```python
from build123d import *

# Parameters (mm, degrees)
BOSS_EXTRUDE1_DEPTH = 37.592
FILLET1_R           = 12.7
FILLET2_R           = 50.8
FILLET3_R           = 12.7
SCALE1_SCALE        = 0.05


with BuildPart() as part:
    # Sketch1 → Boss-Extrude1 (new body)
    with BuildSketch(Plane.XY):
        with BuildLine():
            Line((0, 109.420372667), (250.19, 109.420372667))
            ThreePointArc((250.19, 109.420372667), (267.97, 91.640372667), (250.19, 73.860372667))
            Line((250.19, 73.860372667), (237.49, 73.860372667))
            Line((237.49, 73.860372667), (237.49, 23.060372667))
            Line((237.49, 23.060372667), (250.19, 23.060372667))
            ThreePointArc((250.19, 23.060372667), (267.97, 5.280372667), (250.19, -12.499627333))
            ThreePointArc((250.19, -12.499627333), (146.843102498, -20.027410993), (44.744230284, -37.721168163))
            ThreePointArc((44.744230284, -37.721168163), (-1.227067533, -59.631780483), (17.441932467, -12.25136687))
            ThreePointArc((17.441932467, -12.25136687), (107.033415037, 14.717722357), (200.152, 23.822372667))
            Line((200.152, 23.822372667), (200.152, 72.082372667))
            Line((200.152, 72.082372667), (-75.968392762, 72.082372667))
            Line((-75.968392762, 72.082372667), (-75.968392762, 21.282372667))
            Line((-75.968392762, 21.282372667), (-96.52, 21.282372667))
            Line((-96.52, 21.282372667), (-170.457211488, 45.010876589))
            Line((-170.457211488, 45.010876589), (-170.457211488, 77.522876589))
            Line((-170.457211488, 77.522876589), (-96.52, 53.794372667))
            Line((-96.52, 53.794372667), (-96.52, 139.901603313))
            Line((-96.52, 139.901603313), (-96.52, 160.220372667))
            Line((-96.52, 160.220372667), (0, 160.220372667))
            Line((0, 160.220372667), (0, 109.420372667))
        make_face()
    extrude(amount=BOSS_EXTRUDE1_DEPTH)

    # Fillet1
    fillet1_edges = [part.edges().sort_by_distance(p)[0] for p in [
        (-75.968392762, 21.282372667, 18.796),
    ]]
    fillet(fillet1_edges, radius=FILLET1_R)

    # Fillet2
    fillet2_edges = [part.edges().sort_by_distance(p)[0] for p in [
        (-96.52, 160.220372667, 18.796),
    ]]
    fillet(fillet2_edges, radius=FILLET2_R)

    # Fillet3
    fillet3_edges = [part.edges().sort_by_distance(p)[0] for p in [
        (-96.52, 53.794372667, 18.796),
    ]]
    fillet(fillet3_edges, radius=FILLET3_R)


with BuildPart() as part_1:
    # Scale1: scaled about (66.164273322, 56.765113867, 18.796)
    add(part.part.scale(SCALE1_SCALE).moved(Location((62.856059656, 53.926858174, 17.8562))))


solid = part_1.part
```
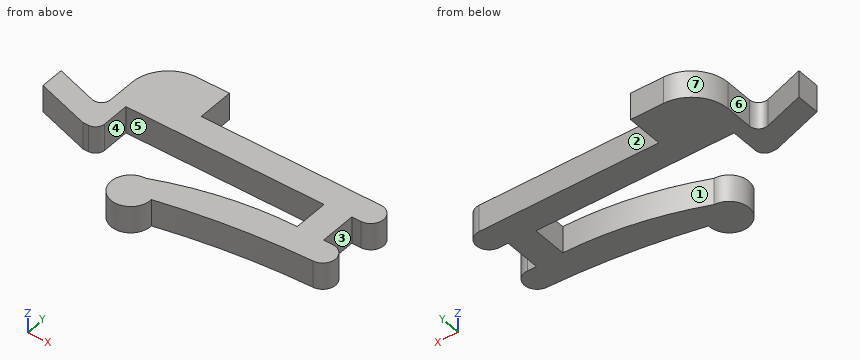
CAD build for the part. Positions are in the model's coordinates, mm. Face numbers are marked on the shaded views. A direction names the side the tool comes from. Give positions to 0.01 mm unless a question says otherwise; leave off trailing zeros. Loops run counter-clockwise (first coordinate to the right, second up) from the corner with the lowest first, then second, coordinate; pieces in that order, holes last. Notation, with made-up numbers: (50, -4) -> (78, -4) arc R15 ccw to (78, 3) -> close; hole circle Ø5 at (-37.75, 77.25). An arc over 180 degrees is marked (long way). Use a Markdown table: item, result.
1. Slice it at A-A (y = 56.5). List the corners of the cut face in (x, z).
Check result:
| item | result |
|---|---|
| outline | (54.33, 17.86) -> (59.06, 17.86) -> (59.06, 19.74) -> (54.33, 19.74) -> close; (72.86, 17.86) -> (74.73, 17.86) -> (74.73, 19.74) -> (72.86, 19.74) -> close |
2. Slice it at C-C (x = 69.5). List the corners of the cut face in (y, z) (3 decimals).
Check result:
| item | result |
|---|---|
| outline | (52.835, 17.856) -> (54.881, 17.856) -> (54.881, 19.736) -> (52.835, 19.736) -> close; (57.531, 17.856) -> (59.398, 17.856) -> (59.398, 19.736) -> (57.531, 19.736) -> close |
3. Which spindle directions (+Z, -Z, +X, -X, +Y, -Y) get a long thin tool onto all of the face, cutting with end or side? Do the marked faces 1, 2, 3 and 4. Say none if no direction does.
Check result:
| item | result |
|---|---|
| face 1 | +Z, -Z |
| face 2 | +Z, -Z, +X, +Y |
| face 3 | +Z, -Z, +X |
| face 4 | +Z, -Z, -Y |
4. Slice it at D-D (y = 51.5). List the corners of the cut face in (x, z), plus the area to 3 significant figures.
Check result:
| item | result |
|---|---|
| outline | (62.43, 17.86) -> (65.02, 17.86) -> (65.02, 19.74) -> (62.43, 19.74) -> close |
| area | 4.86 mm^2 |
5. Flat gauge pins, fed straight in: pin 1 (0.7 mm diameter, centred on x = 75, z = 19, fed in from +Y); pin 2 (0.7 mm diameter, centred on x = 75, z = 19, fed in from -Y); pin 3 (0.6 mm diameter, centred on x = 65.5, z = 19, fed in from -Y). Where does each tip first touch, or does it go through?
Check result:
| item | result |
|---|---|
| pin 1 | stops at y = 59.4 |
| pin 2 | stops at y = 53.28 |
| pin 3 | stops at y = 52.06 |
6. Wall check: L1, parallel to X at y = 59.5, z = 19.3; L2, parallel to Y at x = 69.25, z = 18.9; L3, parallel to Y at x = 65.75, z = 18.75. Give the ranges that are in metal, low to high. Write a range as [from, to].
Check result:
| item | result |
|---|---|
| L1 | x = [58.03, 62.86] |
| L2 | y = [52.8, 54.84], [57.53, 59.4] |
| L3 | y = [52.18, 54.04], [57.53, 59.4] |
7. Mould opens along Y. For the marked faces 5, 6 and 7 say: pulls with the +Y half, pulls with the -Y half, needs draft (parallel to the pull), parting line crosses it, or undercut.
Check result:
| item | result |
|---|---|
| face 5 | undercut |
| face 6 | needs draft |
| face 7 | pulls with the +Y half |
8. Slice it at B-B (z = 18.75). List the corners of the cut face in (x, y) (3 decimals), plus the area to 3 significant figures.
Check result:
| item | result |
|---|---|
| outline | (54.333, 56.177) -> (58.03, 54.991) -> (58.423, 54.991) arc R0.635 ccw to (59.058, 55.626) -> (59.058, 57.531) -> (72.864, 57.531) -> (72.864, 55.118) arc R24.037 ccw to (63.728, 53.314) arc R1.368 ccw (long way) to (65.093, 52.041) arc R52.416 cw to (75.366, 53.302) arc R0.889 ccw to (75.366, 55.08) -> (74.731, 55.08) -> (74.731, 57.62) -> (75.366, 57.62) arc R0.889 ccw to (75.366, 59.398) -> (62.856, 59.398) -> (62.856, 61.938) -> (60.57, 61.938) arc R2.54 ccw to (58.03, 59.398) -> (58.03, 57.487) arc R0.635 cw to (57.201, 56.883) -> (54.333, 57.803) -> close |
| area | 85.6 mm^2 |
